Autodesk Inventor part; units mm, degrees
ref_plane "YZ Plane" through (0, 0, 0) normal (1, 0, 0) x (0, 1, 0)
ref_plane "XZ Plane" through (0, 0, 0) normal (0, 1, 0) x (-1, 0, 0)
ref_plane "XY Plane" through (0, 0, 0) normal (0, 0, 1) x (1, 0, 0)
sketch "Skizze1" plane through (0, 0, 0) normal (0, 1, 0) x (-1, 0, 0)
  line L0 (9.7, -17.018) -> (-9.7, -17.018)
  line L1 (-12.7, -14.018) -> (-12.7, 14.018)
  line L2 (-9.7, 17.018) -> (9.7, 17.018)
  line L3 (12.7, 14.018) -> (12.7, -14.018)
  line L4 (0, -24.695) -> (0, 24.695)
  line L5 (18.6498, 0) -> (-18.6498, 0)
  circle A0 centre (10.16, -14.9291) radius 1.143
  circle A1 centre (-10.16, -14.9291) radius 1.143
  arc A2 (9.7, -17.018) -> (12.7, -14.018) centre (9.7, -14.018) ccw
  arc A3 (-12.7, -14.018) -> (-9.7, -17.018) centre (-9.7, -14.018) ccw
  arc A4 (12.7, 14.018) -> (9.7, 17.018) centre (9.7, 14.018) ccw
  arc A5 (-9.7, 17.018) -> (-12.7, 14.018) centre (-9.7, 14.018) ccw
  line L6 (7.5, -7.5) -> (-7.5, -7.5)
  line L7 (-7.5, -7.5) -> (-7.5, 7.5)
  line L8 (-7.5, 7.5) -> (7.5, 7.5)
  line L9 (7.5, 7.5) -> (7.5, -7.5)
  point P0 (0, 0)
  dimension "d0" = 25.4
  dimension "d1" = 34.036
  dimension "d2" = 2.286
  dimension "d3" = 2.286
  dimension "d4" = 20.32
  dimension "d5" = 3
  dimension "d6" = 3
  dimension "d7" = 3
  dimension "d8" = 3
  dimension "d9" = 15
  dimension "d10" = 15
extrude "Extrusion1" add sketch "Skizze1" along normal blind 1
extrude "Extrusion2" add sketch "Skizze1" along normal blind 5 contours L6 L7 L5 L4 | L4 L5 L9 L6 | L5 L7 L8 L4 | L4 L8 L9 L5
properties part number "GPSSensor"
Could you check a few things on this model? Use its own coordinates, in mm. A direction names the side the tool comes from. Give positions to 0.01 mm unless a question says otherwise; leave off trailing zeros. Loops run counter-clockwise (first coordinate to the right, second up) from the corner with the lowest first, then second, coordinate; pieces in that order, holes last. Notation, with made-up numbers: M 79,64.25 L 133,64.25 A19 ccw 133,81.25 Z; hole C 66.25,34.5 d1. An arc over 180 degrees is marked long. Answer as a JSON object with one key per item and string values.
Q1. Suppose I cut it at D-D, the plane y = 2.75. List the corners of the cut face in (x, z) for me, plus the area to 3 significant figures.
Values found:
{"outline": "M -7.5,-7.5 L 7.5,-7.5 L 7.5,7.5 L -7.5,7.5 Z", "area": "225 mm²"}
Q2. Suppose I cut it at C-C, the plane x = -10.16. List the corners of the cut face in (y, z) for me, plus the area to 3 significant figures.
Values found:
{"outline": "M 0,-16.98 L 1,-16.98 L 1,-16.07 L 0,-16.07 Z; M 0,-13.79 L 1,-13.79 L 1,16.98 L 0,16.98 Z", "area": "31.7 mm²"}
Q3. Suppose I cut it at B-B, the plane z = -5. List the corners of the cut face in (x, y) for me.
Values found:
{"outline": "M -12.7,0 L 12.7,0 L 12.7,1 L 7.5,1 L 7.5,5 L -7.5,5 L -7.5,1 L -12.7,1 Z"}
Q4. For P1, Ø2, axis at y = 3, z = -0.5, coming from the -X side; P2, Ø3.5, axis at x = 10.16, z = -14.93, coming from the +Y side; P3, Ø1.2, axis at x = -3.5, y = 3.5, coming from the -Z side, each with a flat end and sliding along its axis, tell me the tip position at first contact or that it passes through.
Values found:
{"P1": "stops at x = -7.5", "P2": "stops at y = 1", "P3": "stops at z = -7.5"}
Q5. If I drill on probe 1 along Z at (x, y) = (4.25, 1.9); probe 2 along Y at (x, z) = (3.5, 14.5), over which ranges is the centre line in solid material (lowest first)? Write a range as [from, to].
Values found:
{"probe 1": "z = [-7.5, 7.5]", "probe 2": "y = [0, 1]"}
Q6. Suppose I cut it at A-A, the plane x = 4.75. List the corners of the cut face in (y, z) for me.
Values found:
{"outline": "M 0,-17.02 L 1,-17.02 L 1,-7.5 L 5,-7.5 L 5,7.5 L 1,7.5 L 1,17.02 L 0,17.02 Z"}
Q7. For faces 4 (the flat face through (0, 3, -7.5)), 5 (the flat face through (0, 3, 7.5)), 6 (the flat face through (-7.5, 3, 0)), which set-ups out of +Z, -Z, +X, -X, +Y, -Y let a thin tool reach every point of the face, with its end or its side?
Values found:
{"face 4": "-Z, +X, -X, +Y", "face 5": "+Z, +X, -X, +Y", "face 6": "+Z, -Z, -X, +Y"}
Q8. If we mould it in two halves opening along X, with no side actions, what happens to faces 1 (the cylindrical face through (-11.84, 0.49, -16.12)), 2 (the flat face through (7.5, 3, 0)), 3 (the cylindrical face through (11.067, 0.493, -14.234))? For each: pulls with the +X half, pulls with the -X half, needs draft (parallel to the pull), parting line crosses it, or undercut.
Values found:
{"face 1": "pulls with the -X half", "face 2": "pulls with the +X half", "face 3": "undercut"}
